from build123d import *

# Parameters (mm, degrees)
SKETCH1_W           = 210
SKETCH1_H           = 150
BOSS_EXTRUDE1_DEPTH = 115
SKETCH3_W           = 176.973663014
SKETCH3_H           = 90
CUT_EXTRUDE1_DEPTH  = 129
CUT_EXTRUDE2_REACH  = 174.844
SKETCH4_R           = 3.0725
CUT_EXTRUDE3_REACH  = 174.844
SKETCH5_R           = 51.5


with BuildPart() as part:
    # Sketch1 → Boss-Extrude1 (new body)
    with BuildSketch(Plane.XY):
        Rectangle(SKETCH1_W, SKETCH1_H)
    extrude(amount=BOSS_EXTRUDE1_DEPTH)

    # Sketch3 → Cut-Extrude1 (cut)
    with BuildSketch(Plane.XZ.offset(75)):
        with Locations((0, 57.5)):
            Rectangle(SKETCH3_W, SKETCH3_H)
    extrude(amount=-CUT_EXTRUDE1_DEPTH, mode=Mode.SUBTRACT)

    # Sketch4 → Cut-Extrude2 (cut, up to next)
    with BuildSketch(Plane.XY.offset(115), mode=Mode.PRIVATE) as cut_extrude2_sk1:
        with Locations((77.942286341, 43.874821937)):
            Circle(SKETCH4_R)
    cut_extrude2_tool1 = extrude(cut_extrude2_sk1.sketch, amount=-CUT_EXTRUDE2_REACH, mode=Mode.PRIVATE) & part.part
    # Sketch4 → Cut-Extrude2 (cut, up to next)
    with BuildSketch(Plane.XY.offset(115), mode=Mode.PRIVATE) as cut_extrude2_sk2:
        with Locations((-77.942286341, 43.874821937)):
            Circle(SKETCH4_R)
    cut_extrude2_tool2 = extrude(cut_extrude2_sk2.sketch, amount=-CUT_EXTRUDE2_REACH, mode=Mode.PRIVATE) & part.part
    # Sketch4 → Cut-Extrude2 (cut, up to next)
    with BuildSketch(Plane.XY.offset(115), mode=Mode.PRIVATE) as cut_extrude2_sk3:
        with Locations((-77.942286341, -43.874821937)):
            Circle(SKETCH4_R)
    cut_extrude2_tool3 = extrude(cut_extrude2_sk3.sketch, amount=-CUT_EXTRUDE2_REACH, mode=Mode.PRIVATE) & part.part
    # Sketch4 → Cut-Extrude2 (cut, up to next)
    with BuildSketch(Plane.XY.offset(115), mode=Mode.PRIVATE) as cut_extrude2_sk4:
        with Locations((77.942286341, -43.874821937)):
            Circle(SKETCH4_R)
    cut_extrude2_tool4 = extrude(cut_extrude2_sk4.sketch, amount=-CUT_EXTRUDE2_REACH, mode=Mode.PRIVATE) & part.part
    add(cut_extrude2_tool1.solids().sort_by_distance((77.942286, 43.874822, 115))[0], mode=Mode.SUBTRACT)
    add(cut_extrude2_tool2.solids().sort_by_distance((-77.942286, 43.874822, 115))[0], mode=Mode.SUBTRACT)
    add(cut_extrude2_tool3.solids().sort_by_distance((-77.942286, -43.874822, 115))[0], mode=Mode.SUBTRACT)
    add(cut_extrude2_tool4.solids().sort_by_distance((77.942286, -43.874822, 115))[0], mode=Mode.SUBTRACT)

    # Sketch5 → Cut-Extrude3 (cut, up to next)
    with BuildSketch(Plane.XY.offset(115), mode=Mode.PRIVATE) as cut_extrude3_sk1:
        Circle(SKETCH5_R)
    cut_extrude3_tool1 = extrude(cut_extrude3_sk1.sketch, amount=-CUT_EXTRUDE3_REACH, mode=Mode.PRIVATE) & part.part
    add(cut_extrude3_tool1.solids().sort_by_distance((0, 0, 115))[0], mode=Mode.SUBTRACT)


solid = part.part
Geometry: final body of the model. Coordinates: model frame, mm. A direction names the side the tool comes from. Coordinates: 2 decimals unless noted, no trailing zeros. Order: outer loops, then holes, each group sorted by start corner. A loop starts at its lowest first (then second) coordinate and runs counter-clockwise, first axis right, second up.
1) Set-up query: faces 1 (the cylindrical face through (75.5, 42.01, 108.84)), 2 (the flat face through (-1, -54, 102.5)), 3 (the flat face through (-1, -75, 108)). Return all of +Z, -Z, +X, -X, +Y, -Y with unobstructed straight access to the full face (end or side cutting, diameter ignored); none if empty.
Result sheet:
face 1: +Z
face 2: -Y
face 3: +Z, -Z, +X, -X, -Y
2) Draft query along X for faces 4 (the flat face through (105, -1, 57)), 5 (the flat face through (-25, -49, 115)), 6 (the flat face through (-1, 54, 58)). Return one class per face: released by +X, released by -X, zero draft, split by the parting line, or undercut.
Result sheet:
face 4: released by +X
face 5: zero draft
face 6: undercut
3) Ray query, probe 1 along Z at (x, y) = (36, -63); probe 2 along X at (y, z) = (-40, 22); probe 3 along Y at (x, z) = (-81.5, 30). Return the intervals inside material, ascending.
Result sheet:
probe 1: z = 0 to 12.5, 102.5 to 115
probe 2: x = -105 to -88.49, 88.49 to 105
probe 3: y = 54 to 75
4) First-contact query: P1, Ø1.5, axis at x = -33.5, z = 59, coming from the -Y side; P2, Ø5, axis at x = -77.94, y = -43.87, coming from the -Z side; P3, Ø3.5, axis at x = 77.94, y = 43.87, coming from the +Z side. Flat tips, straight axial feed; report the tip coordinate or a pass-through.
Result sheet:
P1: stops at y = 54
P2: stops at z = 0
P3: stops at z = 12.5
5) Section B-B (z = 15). Return loops of the section in (x, y).
Result sheet:
outline: (-105, -75) - (-88.49, -75) - (-88.49, 54) - (88.49, 54) - (88.49, -75) - (105, -75) - (105, 75) - (-105, 75) - close
6) Section A-A (x = 0). Return loops of the section in (y, z), then the cut area to 3 significant figures.
Result sheet:
outline: (-75, 0) - (75, 0) - (75, 115) - (51.5, 115) - (51.5, 102.5) - (54, 102.5) - (54, 12.5) - (-75, 12.5) - close; (-75, 102.5) - (-51.5, 102.5) - (-51.5, 115) - (-75, 115) - close
area: 4,350 mm2
7) Section C-C (y = 0). Return loops of the section in (x, z), then the cut area to 3 significant figures.
Result sheet:
outline: (-105, 0) - (105, 0) - (105, 115) - (51.5, 115) - (51.5, 102.5) - (88.49, 102.5) - (88.49, 12.5) - (-88.49, 12.5) - (-88.49, 102.5) - (-51.5, 102.5) - (-51.5, 115) - (-105, 115) - close
area: 6,930 mm2
8) Section D-D (x = -38). Return loops of the section in (y, z).
Result sheet:
outline: (-75, 0) - (75, 0) - (75, 115) - (34.76, 115) - (34.76, 102.5) - (54, 102.5) - (54, 12.5) - (-75, 12.5) - close; (-75, 102.5) - (-34.76, 102.5) - (-34.76, 115) - (-75, 115) - close
